For this review, use the dimensioned drawing (mm, ordinates from the lowest corner) and the shaded views. Give positions to 0.01 mm unless a question says otherwise; leave off trailing zeros. Loops run counter-clockwise (first coordinate to the right, second up) from the corner with the lowest first, then second, coordinate; pieces in that order, holes last. Notation, with made-up numbers: (-15, 89.25) -> (24, 89.25) arc R35 cw to (24, 125.25) -> close; hole circle Ø7 at (40.5, 75). An arc over 180 degrees is marked (long way). Use a Markdown table: item, result. Add a question column.
1. Add section C-C (x = 41.5). State the section outline as (y, z) points.
2. Add section D-D (z = 13.5). State the section outline as (x, y) points (1 decimal), and give its area (3 significant figures).
3. Add section A-A (x = 12.7). State the section outline as (y, z) points (1 decimal).
4. To check wall thickness, follow line 1 (X direction, y = 1.25, z = 23.5) (1 decimal); line 2 (X direction, y = 1.9, z = 28) (1 decimal); line 3 (X direction, y = 1.9, z = 6) (1 decimal). State the ranges of each line that lie inside material, in increasing order.
5. For pin 1 Ø2 at (x, z) = (49.9, 5.22) entering from -Y; pin 2 Ø3 at (x, z) = (57.52, 18.42) entering from +Y; pin 3 Ø0.9 at (x, y) = (17.5, 1) entering from -Z (3 decimals), all flat-tipped, find the tip position at first contact; note any pin that passes through.
6. Add section B-B (y = 1.5). Count the separate pieces of the cut face and the enclosed holes in it, and give its area (3 significant figures).
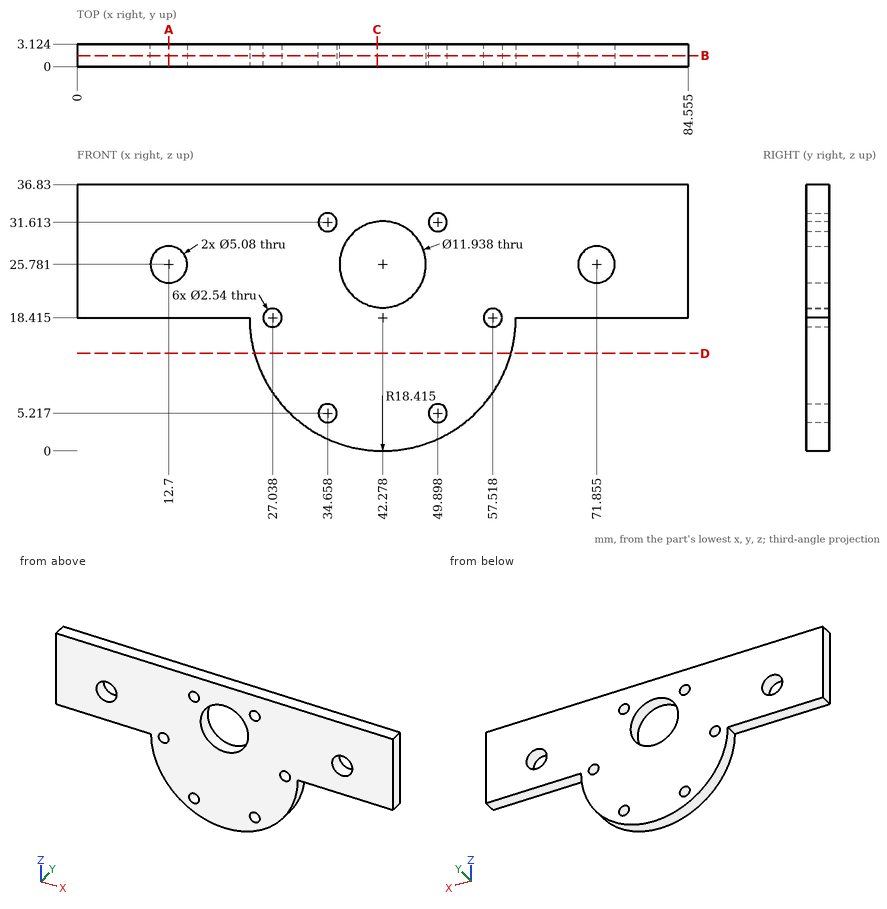
Taken from the geometry:
| question | item | result |
|---|---|---|
| 1 | outline | (0, 0.02) -> (3.12, 0.02) -> (3.12, 19.86) -> (0, 19.86) -> close; (0, 31.7) -> (3.12, 31.7) -> (3.12, 36.83) -> (0, 36.83) -> close |
| 2 | outline | (24.5, 0) -> (60, 0) -> (60, 3.1) -> (24.5, 3.1) -> close |
| 2 | area | 111 mm^2 |
| 3 | outline | (0, 18.4) -> (3.1, 18.4) -> (3.1, 23.2) -> (0, 23.2) -> close; (0, 28.3) -> (3.1, 28.3) -> (3.1, 36.8) -> (0, 36.8) -> close |
| 4 | line 1 | x = 0 to 11.6, 13.8 to 36.8, 47.8 to 70.7, 73 to 84.6 |
| 4 | line 2 | x = 0 to 11.5, 13.9 to 36.7, 47.8 to 70.6, 73.1 to 84.6 |
| 4 | line 3 | x = 28.7 to 33.7, 35.7 to 48.9, 50.9 to 55.9 |
| 5 | pin 1 | passes through |
| 5 | pin 2 | stops at y = 3.12 |
| 5 | pin 3 | stops at z = 18.415 |
| 6 | separate pieces | 1 |
| 6 | enclosed holes | 9 |
| 6 | area | 1,910 mm^2 |
